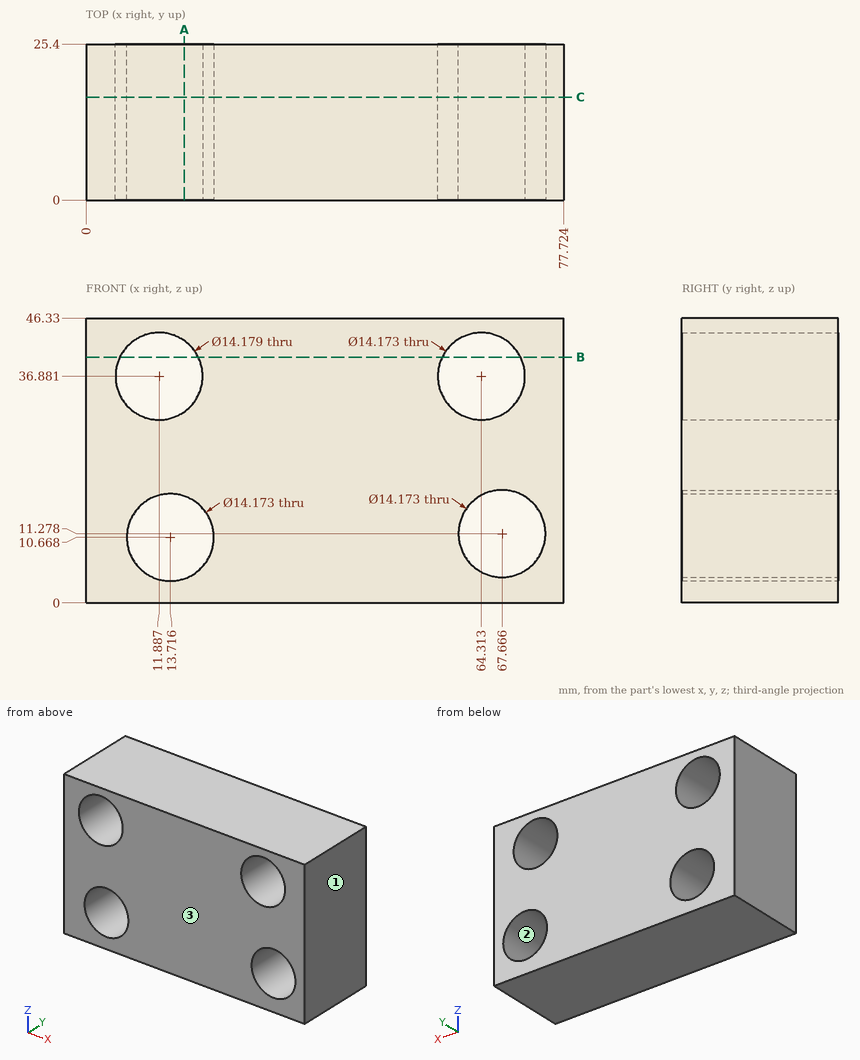
Here's the drawing with two shaded views (mm, measured from the low corner). I have some questions. Round coordinates to 2 decimals unless told otherwise and drop trailing zeros. Loops run counter-clockwise (first coordinate to the right, second up) from the corner with the lowest first, then second, coordinate; pieces in that order, holes last.
Item 1: Please list where these lines run through material, in increasing order: L1, parallel to X at y = 12.5, z = 36 (1 decimal); L2, parallel to X at y = 1.75, z = 41.5 (1 decimal); L3, parallel to Z at x = 17, y = 1.75.
Item 2: Suppose I cut it at C-C, the plane y = 16.75. Write out the boundary of the cut face in (x, z) (1 decimal), then the cut area to 3 significant figures.
Item 3: Will this pin go through, and if not, where does the flat tip stop? pin 1 Ø12 at (y, z) = (7, 29.5) entering from -X.
Item 4: Suppose I cut it at A-A, the plane x = 16. Write out the boundary of the cut face in (y, z) (1 decimal).
Item 5: Suppose I cut it at B-B, the plane z = 40. Write out the boundary of the cut face in (x, y), then the cut area to 3 significant figures.
Item 6: If we mould it in two halves opening along X, with no side actions, what happens to the marked faces 1, 2 and 3? For each: +X half, -X half, draft (parallel to the pull), parting line (faces both ways), or undercut.
Reported:
1. L1: x = 0 to 4.9, 18.9 to 57.3, 71.3 to 77.7
1. L2: x = 0 to 6.5, 17.3 to 58.9, 69.7 to 77.7
1. L3: z = 0 to 4.39, 16.95 to 31.97, 41.79 to 46.33
2. outline: (0, 0) - (77.7, 0) - (77.7, 46.3) - (0, 46.3) - close; hole circle Ø14.2 at (11.9, 36.9); hole circle Ø14.2 at (13.7, 10.7); hole circle Ø14.2 at (64.3, 36.9); hole circle Ø14.2 at (67.7, 11.3)
2. area: 2,970 mm2
3. pin 1: stops at x = 0
4. outline: (0, 0) - (25.4, 0) - (25.4, 4) - (0, 4) - close; (0, 17.4) - (25.4, 17.4) - (25.4, 31.1) - (0, 31.1) - close; (0, 42.7) - (25.4, 42.7) - (25.4, 46.3) - (0, 46.3) - close
5. outline: (0, 0) - (5.52, 0) - (5.52, 25.4) - (0, 25.4) - close; (18.25, 0) - (57.95, 0) - (57.95, 25.4) - (18.25, 25.4) - close; (70.68, 0) - (77.72, 0) - (77.72, 25.4) - (70.68, 25.4) - close
5. area: 1,330 mm2
6. face 1: +X half
6. face 2: undercut
6. face 3: draft
